from build123d import *

# Parameters (mm, degrees)
F0_W     = 63.5
F0_H     = 63.5
F0_R     = 25.2984
F0_R_2   = 19.0754
F1_DEPTH = 5.969
F3_R     = 25.2984
F3_R_2   = 19.0754
F4_DEPTH = 1.651
F5_D     = 5.08


with BuildPart() as f1:
    # F0 (on Front) → F1 (new body)
    with BuildSketch(Plane.XZ):
        with Locations((31.75, 31.75)):
            Rectangle(F0_W, F0_H)
        with Locations((31.75, 31.75)):
            Circle(F0_R, mode=Mode.SUBTRACT)
        with Locations((31.75, 31.75)):
            Circle(F0_R)
        with Locations((31.75, 31.75)):
            Circle(F0_R_2, mode=Mode.SUBTRACT)
        with Locations((31.75, 31.75)):
            Circle(F0_R_2)
    extrude(amount=F1_DEPTH)

    # F3 (on face) → F4 (cut)
    with BuildSketch(Plane.XZ.offset(5.969)):
        with Locations((31.75, 31.75)):
            Circle(F3_R)
        with Locations((31.75, 31.75)):
            Circle(F3_R_2, mode=Mode.SUBTRACT)
    extrude(amount=-F4_DEPTH, mode=Mode.SUBTRACT)

    # F5 (through all)
    with Locations(Plane(origin=(0, 0, 0), x_dir=(1, 0, 0), z_dir=(0, 1, 0))):
        with Locations((10.5156, -52.9971), (52.9971, -52.9971), (10.5156, -10.5156), (52.9971, -10.5156), (31.75, -31.75)):
            Hole(F5_D / 2)


solid = f1.part
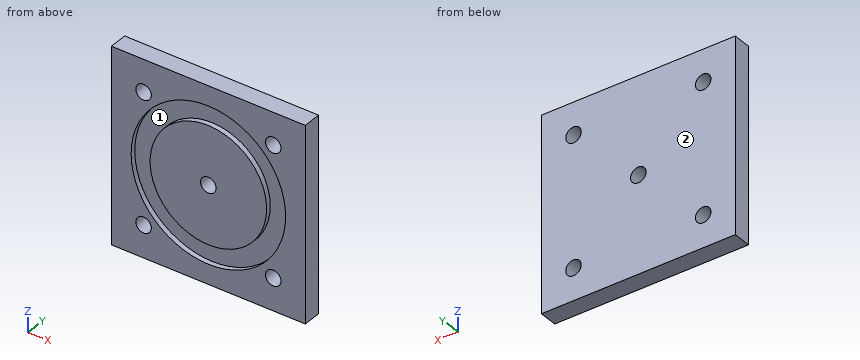
Could you check a few things on this model? Use its own coordinates, in mm. Face numbers are marked on the shaded views. Give positions to 0.01 mm unless a question says otherwise; leave off trailing zeros. Write each loop counter-clockwise with the first axis right and the second up, starting at its lowest first coordinate (ties: lowest second). Pieces come first, ordered by that corner, then holes. Notation, with made-up numbers: (0, 56.25) -> (23, 56.25) arc R19 cw to (23, 74.25) -> close; hole circle Ø9 at (63, 81.25). An arc over 180 degrees is marked (long way). Answer as CSV lines item,"result". Start each with the question number.
(1) I'm going to push a flat-ended pin straight in: pin 1 Ø2 at (y, z) = (-4, 14) entering from -X. Where does the tip first touch, or does it pass through?
(2) If we section it at A-A, the plane z = 31.75: Write out the boundary of the cut face in (x, y), and give its area (3 significant figures).
(3) If we section it at C-C, the plane y = -2.9: Write out the boundary of the cut face in (x, z).
(4) Please list where these lines run through material, in increasing order: line 1 (Z direction, x = 31.75, y = -1.2); line 2 (X direction, y = -4.25, z = 9.5); line 3 (Z direction, x = 51, y = -1.95).
(5) If we mould it in two halves opening along X, with no side actions, what happens to the marked faces 1 and 2? For each: +X half, -X half, draft (parallel to the pull), parting line (faces both ways), or undercut.
(6) If we section it at D-D, the plane x = 9.5: Write out the boundary of the cut face in (y, z).
(7) If we section it at B-B, the plane x = 31.75: Write out the boundary of the cut face in (y, z).
Answer list:
1,pin 1,"x = 0"
2,outline,"(0, -5.97) -> (6.45, -5.97) -> (6.45, -4.32) -> (12.67, -4.32) -> (12.67, -5.97) -> (29.21, -5.97) -> (29.21, 0) -> (0, 0) -> close; (34.29, -5.97) -> (50.83, -5.97) -> (50.83, -4.32) -> (57.05, -4.32) -> (57.05, -5.97) -> (63.5, -5.97) -> (63.5, 0) -> (34.29, 0) -> close"
2,area,"328 mm^2"
3,outline,"(0, 0) -> (63.5, 0) -> (63.5, 63.5) -> (0, 63.5) -> close; hole circle Ø5.08 at (10.52, 10.52); hole circle Ø5.08 at (10.52, 53); hole circle Ø5.08 at (31.75, 31.75); hole circle Ø5.08 at (53, 10.52); hole circle Ø5.08 at (53, 53)"
4,line 1,"0 to 29.21, 34.29 to 63.5"
4,line 2,"0 to 8.19, 12.84 to 50.67, 55.33 to 63.5"
4,line 3,"0 to 8.95, 12.09 to 51.43, 54.57 to 63.5"
5,face 1,"undercut"
5,face 2,"draft"
6,outline,"(-5.97, 0) -> (0, 0) -> (0, 8.19) -> (-5.97, 8.19) -> close; (-5.97, 12.84) -> (0, 12.84) -> (0, 50.67) -> (-5.97, 50.67) -> (-5.97, 43.79) -> (-4.32, 43.79) -> (-4.32, 19.71) -> (-5.97, 19.71) -> close; (-5.97, 55.33) -> (0, 55.33) -> (0, 63.5) -> (-5.97, 63.5) -> close"
7,outline,"(-5.97, 0) -> (0, 0) -> (0, 29.21) -> (-5.97, 29.21) -> (-5.97, 12.67) -> (-4.32, 12.67) -> (-4.32, 6.45) -> (-5.97, 6.45) -> close; (-5.97, 34.29) -> (0, 34.29) -> (0, 63.5) -> (-5.97, 63.5) -> (-5.97, 57.05) -> (-4.32, 57.05) -> (-4.32, 50.83) -> (-5.97, 50.83) -> close"
